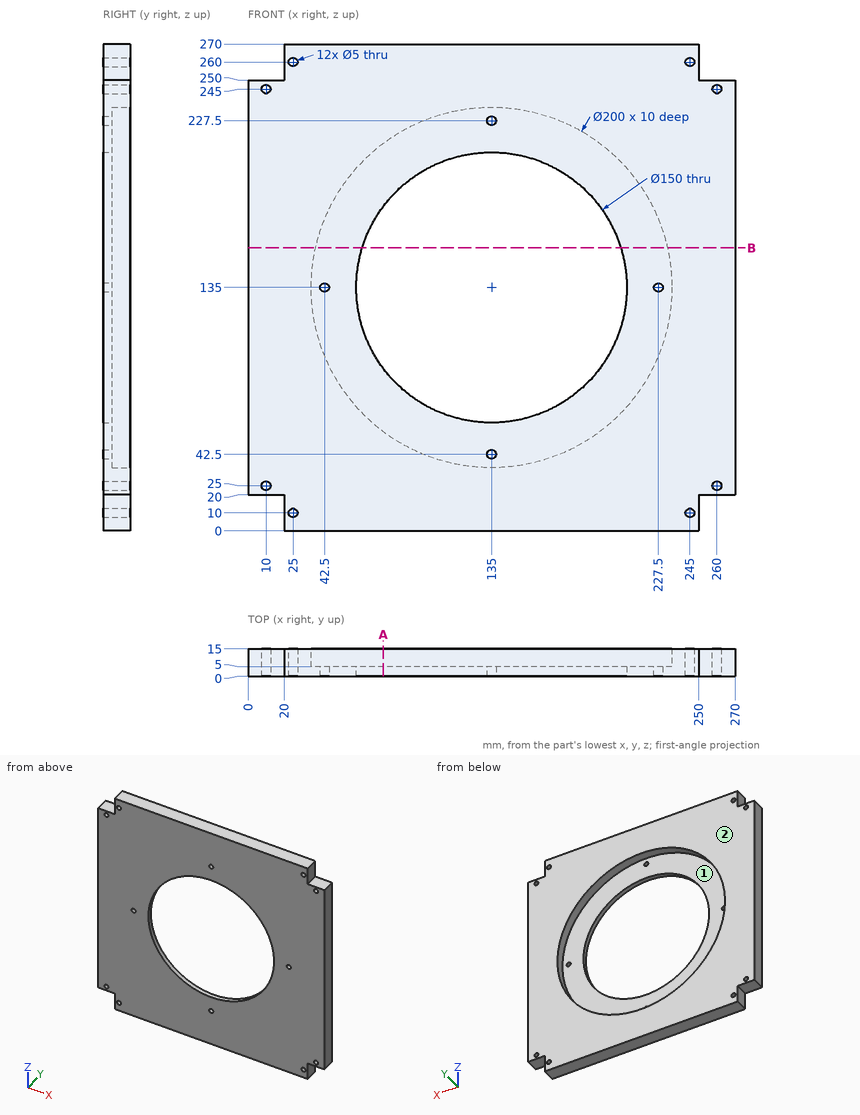
Source: three-view drawing plus pictorial views. Frame: mm from the lowest corner of the part. Coordinates: 2 decimals unless noted, no trailing zeros. Order: outer loops, then holes, each group sorted by start corner. A loop starts at its lowest first (then second) coordinate and runs counter-clockwise, first axis right, second up. Notation, with made-up numbers: (43.5, 1.25) -> (98.5, 1.25) arc R29 ccw to (98.5, 31.25) -> close; hole circle Ø1 at (71.25, 12). An arc over 180 degrees is marked (long way). Write item = value, one per line.
(1) Pull-direction query (Z, two-part tool) for the marked faces 1 and 2; classes: pulls with the +Z half, pulls with the -Z half, needs draft (parallel to the pull), parting line crosses it, or undercut.
Solved:
face_1 = undercut
face_2 = needs draft
(2) Cut plane B-B on z = 157. Return loops of the section in (x, y), plus the area to 3 significant figures.
Solved:
outline = (0, 0) -> (63.3, 0) -> (63.3, 5) -> (37.45, 5) -> (37.45, 15) -> (0, 15) -> close; (206.7, 0) -> (270, 0) -> (270, 15) -> (232.55, 15) -> (232.55, 5) -> (206.7, 5) -> close
area = 1,380 mm²
(3) Line query: line 1 (Z direction, x = 260, y = 11.75); line 2 (X direction, y = 9.25, z = 25). Output: solid intervals per line, ascending.
Solved:
line_1 = 20 to 22.5, 27.5 to 242.5, 247.5 to 250
line_2 = 0 to 7.5, 12.5 to 257.5, 262.5 to 270
(4) Pin query (flat end, axial travel): pin 1 Ø4 at (x, z) = (10, 25) entering from -Y; pin 2 Ø6 at (x, z) = (42.5, 135) entering from +Y; pin 3 Ø4.5 at (x, y) = (264, 10) entering from -Z. Return the tip coordinate at first contact, or that it passes through.
Solved:
pin_1 = through
pin_2 = 5
pin_3 = 20
(5) Cut plane A-A on x = 75. Return loops of the section in (y, z), plus the area to 3 significant figures.
Solved:
outline = (0, 0) -> (15, 0) -> (15, 55) -> (5, 55) -> (5, 90) -> (0, 90) -> close; (0, 180) -> (5, 180) -> (5, 215) -> (15, 215) -> (15, 270) -> (0, 270) -> close
area = 2,000 mm²
